```python
from build123d import *

# Parameters (mm, degrees)
SKETCH1_W           = 50
SKETCH1_H           = 60
BOSS_EXTRUDE1_DEPTH = 10
SKETCH2_R           = 1.5
CUT_EXTRUDE1_DEPTH  = 6
CUT_EXTRUDE2_REACH  = 41.509
SKETCH3_R           = 3
SKETCH5_W           = 25
SKETCH5_H           = 6
BOSS_EXTRUDE3_DEPTH = 30
CUT_EXTRUDE3_REACH  = 78.322
SKETCH6_W           = 22
SKETCH6_H           = 19.25
SKETCH7_R           = 1
CUT_EXTRUDE4_DEPTH  = 2.5
CUT_EXTRUDE5_REACH  = 75.602
SKETCH8_R           = 2
BOSS_EXTRUDE4_DEPTH = 5
CHAMFER1_SIZE       = 7.5
CHAMFER2_SIZE       = 10
CHAMFER4_SIZE       = 6.5
CHAMFER5_SIZE       = 4
CHAMFER6_SIZE       = 4
CHAMFER7_SIZE       = 2


# Some blends are built 0.0001 mm under size
with BuildPart() as part:
    # Sketch1 → Boss-Extrude1 (new body)
    with BuildSketch(Plane(origin=(0, 0, 0), x_dir=(1, 0, 0), z_dir=(0, 1, 0))):
        Rectangle(SKETCH1_W, SKETCH1_H)
    extrude(amount=BOSS_EXTRUDE1_DEPTH)

    # Sketch2 → Cut-Extrude1 (cut)
    with BuildSketch(Plane(origin=(0, 0, 0), x_dir=(1, 0, 0), z_dir=(0, 1, 0))):
        with Locations(Location((-21, 7.7, 0), (0, 0, 270))):
            Circle(SKETCH2_R)
        with Locations(Location((-21, -23, 0), (0, 0, 270))):
            Circle(SKETCH2_R)
        with Locations(Location((21, 7.7, 0), (0, 0, 270))):
            Circle(SKETCH2_R)
        with Locations(Location((21, -23, 0), (0, 0, 270))):
            Circle(SKETCH2_R)
    extrude(amount=CUT_EXTRUDE1_DEPTH, mode=Mode.SUBTRACT)

    # Sketch3 → Cut-Extrude2 (cut, up to next)
    with BuildSketch(Plane.XZ.offset(-6), mode=Mode.PRIVATE) as cut_extrude2_sk1:
        with Locations(Location((-21, 23, 0), (0, 0, 270))):
            Circle(SKETCH3_R)
    cut_extrude2_tool1 = extrude(cut_extrude2_sk1.sketch, amount=-CUT_EXTRUDE2_REACH, mode=Mode.PRIVATE) & part.part
    # Sketch3 → Cut-Extrude2 (cut, up to next)
    with BuildSketch(Plane.XZ.offset(-6), mode=Mode.PRIVATE) as cut_extrude2_sk2:
        with Locations(Location((21, 23, 0), (0, 0, 270))):
            Circle(SKETCH3_R)
    cut_extrude2_tool2 = extrude(cut_extrude2_sk2.sketch, amount=-CUT_EXTRUDE2_REACH, mode=Mode.PRIVATE) & part.part
    # Sketch3 → Cut-Extrude2 (cut, up to next)
    with BuildSketch(Plane.XZ.offset(-6), mode=Mode.PRIVATE) as cut_extrude2_sk3:
        with Locations(Location((21, -7.7, 0), (0, 0, 270))):
            Circle(SKETCH3_R)
    cut_extrude2_tool3 = extrude(cut_extrude2_sk3.sketch, amount=-CUT_EXTRUDE2_REACH, mode=Mode.PRIVATE) & part.part
    # Sketch3 → Cut-Extrude2 (cut, up to next)
    with BuildSketch(Plane.XZ.offset(-6), mode=Mode.PRIVATE) as cut_extrude2_sk4:
        with Locations(Location((-21, -7.7, 0), (0, 0, 270))):
            Circle(SKETCH3_R)
    cut_extrude2_tool4 = extrude(cut_extrude2_sk4.sketch, amount=-CUT_EXTRUDE2_REACH, mode=Mode.PRIVATE) & part.part
    add(cut_extrude2_tool1.solids().sort_by_distance((-21, 6, 23))[0], mode=Mode.SUBTRACT)
    add(cut_extrude2_tool2.solids().sort_by_distance((21, 6, 23))[0], mode=Mode.SUBTRACT)
    add(cut_extrude2_tool3.solids().sort_by_distance((21, 6, -7.7))[0], mode=Mode.SUBTRACT)
    add(cut_extrude2_tool4.solids().sort_by_distance((-21, 6, -7.7))[0], mode=Mode.SUBTRACT)

    # Sketch5 → Boss-Extrude3 (add)
    with BuildSketch(Plane(origin=(0, 10, 0), x_dir=(1, 0, 0), z_dir=(0, 1, 0))):
        with Locations((0, 27)):
            Rectangle(SKETCH5_W, SKETCH5_H)
    extrude(amount=BOSS_EXTRUDE3_DEPTH)

    # Sketch6 → Cut-Extrude3 (cut, up to next)
    with BuildSketch(Plane(origin=(0, 0, -30), x_dir=(-1, 0, 0), z_dir=(0, 0, -1)), mode=Mode.PRIVATE) as cut_extrude3_sk1:
        with Locations((0, 24.625)):
            Rectangle(SKETCH6_W, SKETCH6_H)
    cut_extrude3_tool1 = extrude(cut_extrude3_sk1.sketch, amount=-CUT_EXTRUDE3_REACH, mode=Mode.PRIVATE) & part.part
    add(cut_extrude3_tool1.solids().sort_by_distance((0, 24.625, -30))[0], mode=Mode.SUBTRACT)

    # Sketch7 → Cut-Extrude4 (cut)
    with BuildSketch(Plane.XY.offset(-24)):
        with Locations((10.25, 12.25)):
            Circle(SKETCH7_R)
        with Locations((-10.25, 12.25)):
            Circle(SKETCH7_R)
        with Locations((-10.25, 36.7)):
            Circle(SKETCH7_R)
        with Locations((10.25, 36.7)):
            Circle(SKETCH7_R)
    extrude(amount=-CUT_EXTRUDE4_DEPTH, mode=Mode.SUBTRACT)

    # Sketch8 → Cut-Extrude5 (cut, up to next)
    with BuildSketch(Plane.XY.offset(-26.5), mode=Mode.PRIVATE) as cut_extrude5_sk1:
        with Locations((-10.25, 36.7)):
            Circle(SKETCH8_R)
    cut_extrude5_tool1 = extrude(cut_extrude5_sk1.sketch, amount=-CUT_EXTRUDE5_REACH, mode=Mode.PRIVATE) & part.part
    # Sketch8 → Cut-Extrude5 (cut, up to next)
    with BuildSketch(Plane.XY.offset(-26.5), mode=Mode.PRIVATE) as cut_extrude5_sk2:
        with Locations((10.25, 36.7)):
            Circle(SKETCH8_R)
    cut_extrude5_tool2 = extrude(cut_extrude5_sk2.sketch, amount=-CUT_EXTRUDE5_REACH, mode=Mode.PRIVATE) & part.part
    # Sketch8 → Cut-Extrude5 (cut, up to next)
    with BuildSketch(Plane.XY.offset(-26.5), mode=Mode.PRIVATE) as cut_extrude5_sk3:
        with Locations((10.25, 12.25)):
            Circle(SKETCH8_R)
    cut_extrude5_tool3 = extrude(cut_extrude5_sk3.sketch, amount=-CUT_EXTRUDE5_REACH, mode=Mode.PRIVATE) & part.part
    # Sketch8 → Cut-Extrude5 (cut, up to next)
    with BuildSketch(Plane.XY.offset(-26.5), mode=Mode.PRIVATE) as cut_extrude5_sk4:
        with Locations((-10.25, 12.25)):
            Circle(SKETCH8_R)
    cut_extrude5_tool4 = extrude(cut_extrude5_sk4.sketch, amount=-CUT_EXTRUDE5_REACH, mode=Mode.PRIVATE) & part.part
    add(cut_extrude5_tool1.solids().sort_by_distance((-10.25, 36.7, -26.5))[0], mode=Mode.SUBTRACT)
    add(cut_extrude5_tool2.solids().sort_by_distance((10.25, 36.7, -26.5))[0], mode=Mode.SUBTRACT)
    add(cut_extrude5_tool3.solids().sort_by_distance((10.25, 12.25, -26.5))[0], mode=Mode.SUBTRACT)
    add(cut_extrude5_tool4.solids().sort_by_distance((-10.25, 12.25, -26.5))[0], mode=Mode.SUBTRACT)

    # Sketch9 → Boss-Extrude4 (add)
    with BuildSketch(Plane(origin=(12.5, 0, 0), x_dir=(0, 0, -1), z_dir=(1, 0, 0))):
        Polygon((30, 40), (24, 40), (-6, 10), (30, 10), align=None)
    boss_extrude4 = extrude(amount=BOSS_EXTRUDE4_DEPTH)

    # Mirror1: Boss-Extrude4 across plane
    add(boss_extrude4.mirror(Plane(origin=(0, 0, 0), x_dir=(0, 0, 1), z_dir=(1, 0, 0))))

    # Chamfer1
    # the kernel refuses this chamfer: 7.5 mm, written as the material it adds along each edge
    with BuildSketch(Plane(origin=(17.5, 10, 25.28762241), x_dir=(-0.02749587661058632, 0.9996219169112968, 0), z_dir=(0, 0, -1))) as chamfer1_piece_1_section:
        Polygon((CHAMFER1_SIZE * 0.999621916911, CHAMFER1_SIZE * 0.0274958766106), (-CHAMFER1_SIZE * 0.0274958766106, CHAMFER1_SIZE * 0.999621916911), (0, 0), align=None)
    chamfer1_piece_1 = extrude(amount=55.28762241, mode=Mode.PRIVATE)
    chamfer1_piece_1 = split(chamfer1_piece_1, bisect_by=Plane(origin=(19.963540821, 21.141387269, -5.141387269), z_dir=(0, -0.7071067811865512, -0.7071067811865438)), keep=Keep.TOP, mode=Mode.PRIVATE)
    chamfer1_piece_1 = chamfer1_piece_1 - Plane(origin=(21, 12.394681138, -7.7), x_dir=(0, 0, -1), z_dir=(0, -1, 0)) * Cylinder(3, 141, mode=Mode.PRIVATE)
    chamfer1_piece_1 = split(chamfer1_piece_1, bisect_by=Plane(origin=(25, 12.394681138, -13.888093401), z_dir=(-1, 0, 0)), keep=Keep.TOP, mode=Mode.PRIVATE)
    add(chamfer1_piece_1)
    with BuildSketch(Plane(origin=(-17.5, 10, 25.28762241), x_dir=(0.02749587661058632, 0.9996219169112968, 0), z_dir=(0, 0, -1))) as chamfer1_piece_2_section:
        Polygon((CHAMFER1_SIZE * 0.999621916911, -CHAMFER1_SIZE * 0.0274958766106), (-CHAMFER1_SIZE * 0.0274958766106, -CHAMFER1_SIZE * 0.999621916911), (0, 0), align=None)
    chamfer1_piece_2 = extrude(amount=55.28762241, mode=Mode.PRIVATE)
    chamfer1_piece_2 = split(chamfer1_piece_2, bisect_by=Plane(origin=(-19.963548268, 21.141369022, -5.141369022), z_dir=(0, -0.7071067811865512, -0.7071067811865438)), keep=Keep.TOP, mode=Mode.PRIVATE)
    chamfer1_piece_2 = chamfer1_piece_2 - Plane(origin=(-21, 12.394672857, -7.7), x_dir=(0, 0, -1), z_dir=(0, -1, 0)) * Cylinder(3, 141, mode=Mode.PRIVATE)
    chamfer1_piece_2 = split(chamfer1_piece_2, bisect_by=Plane(origin=(-25, 12.394672857, -13.888065186), z_dir=(1, 0, 0)), keep=Keep.TOP, mode=Mode.PRIVATE)
    add(chamfer1_piece_2)

    # Chamfer2
    chamfer2_edges = [part.edges().sort_by_distance(p)[0] for p in [
        (-25, 5, -30),
        (25, 5, -30),
    ]]
    chamfer(chamfer2_edges, length=CHAMFER2_SIZE)

    # Chamfer4
    chamfer4_edges = [part.edges().sort_by_distance(p)[0] for p in [
        (0, 0, -30),
    ]]
    chamfer(chamfer4_edges, length=CHAMFER4_SIZE)

    # Chamfer5
    chamfer5_edges = [part.edges().sort_by_distance(p)[0] for p in [
        (17.5, 40, -25.75),
        (-17.5, 40, -25.75),
    ]]
    chamfer(chamfer5_edges, length=CHAMFER5_SIZE)

    # Chamfer6
    chamfer6_edges = [part.edges().sort_by_distance(p)[0] for p in [
        (0, 10, 30),
    ]]
    chamfer(chamfer6_edges, length=CHAMFER6_SIZE - 0.0001)  # a hair under: the kernel refuses the full size

    # Chamfer7
    chamfer7_edges = [part.edges().sort_by_distance(p)[0] for p in [
        (-11, 34.25, -27),
        (-11, 15, -27),
        (11, 15, -27),
        (11, 34.25, -27),
    ]]
    chamfer(chamfer7_edges, length=CHAMFER7_SIZE)


solid = part.part
```
Can you work these out from the model? Positions are in its coordinate system, mm. A direction names the side the tool comes from. Give positions to 0.01 mm unless a question says otherwise; leave off trailing zeros. Loops run counter-clockwise (first coordinate to the right, second up) from the corner with the lowest first, then second, coordinate; pieces in that order, holes last. Notation, with made-up numbers: M 55,68.5 L 98,68.5 A26 cw 98,107.5 Z; hole C 8.5,45 d11. An arc over 180 degrees is marked long. Use CSV: the item, a comma, the result in double quotes. Start each with the question number.
1. Imagine slicing it at A-A, the plane y = 27.5. Write out the boundary of the cut face in (x, z), plus the area to 3 significant figures.
2. For P1, Ø6.5, axis at y = 25, z = -26.5, coming from the -X side; P2, Ø2.5, axis at x = 10.25, y = 36.7, coming from the -Z side; P3, Ø6, axis at y = 16, z = -13, coming from the +X side, each with a flat end and sliding along its axis, tell me the tip position at first contact or that it passes through.
3. If we mould it in two halves opening along Z, with no side actions, what happens to faces 1 (the face through (-10, 38, -26.5)), 2 (the face through (-18.026, 10.228, -7.309)), 3 (the face through (0, 15, -27)), 4 (the face through (-19.513, 2.958, -7.895))? For each: released by +Z, released by -Z, zero draft, split by the parting line, or undercut.
4. Imagine slicing it at D-D, the plane y = 33.5. Write out the boundary of the cut face in (x, z), plus the area to 3 significant figures.
5. Imagine slicing it at C-C, the plane z = 23. Write out the boundary of the cut face in (x, y), plus the area to 3 significant figures.
6. Imagine slicing it at B-B, the plane x = 7.5. Write out the boundary of the cut face in (y, z).
7. On a 3-axis mill with a long thin cutter (end or side, diameter ignored), from which of +Z, -Z, +X, -X, +Y, -Y can I reach the whole of each face in a straight line? I mean faces 5 (the face through (0, 10, 6)), 6 (the face through (-17.5, 25, -17)), 7 (the face through (-10.01, 33.24, -27.04)), 8 (the face through (9, 12, -26.5)). Say none if no direction works.
8. If I drill on L1, parallel to X at y = 35, z = -23.5; L2, parallel to X at y = 2, z = 23; L3, parallel to Z at x = -8.5, y = 14.5, over which ranges is the centre line in solid material (lowest first)?
Response values:
1,outline,"M -17.5,-27.5 L -15,-30 L -11,-30 L -11,-24 L -12.5,-24 L -12.5,-11.5 L -17.5,-11.5 Z; M 11,-30 L 15,-30 L 17.5,-27.5 L 17.5,-11.5 L 12.5,-11.5 L 12.5,-24 L 11,-24 Z"
1,area,"197 mm^2"
2,P1,"x = -17.5"
2,P2,"z = -26.5"
2,P3,"x = 22"
3,face 1,"released by -Z"
3,face 2,"undercut"
3,face 3,"zero draft"
3,face 4,"undercut"
4,outline,"M -17.5,-27.5 L -15,-30 L -9.75,-30 L -9.75,-24 L -12.5,-24 L -12.5,-17.5 L -17.5,-17.5 Z; M 9.75,-30 L 15,-30 L 17.5,-27.5 L 17.5,-17.5 L 12.5,-17.5 L 12.5,-24 L 9.75,-24 Z"
4,area,"152 mm^2"
5,outline,"M -25,0 L -22.5,0 L -22.5,6 L -24,6 L -24,10 L -25,10 Z; M -19.5,0 L 19.5,0 L 19.5,6 L 18,6 L 18,10 L -18,10 L -18,6 L -19.5,6 Z; M 22.5,0 L 25,0 L 25,10 L 24,10 L 24,6 L 22.5,6 Z"
5,area,"416 mm^2"
6,outline,"M 0,-23.5 L 6.5,-30 L 15,-30 L 15,-24 L 10,-24 L 10,26 L 6,30 L 0,30 Z; M 34.25,-30 L 40,-30 L 40,-24 L 34.25,-24 Z"
7,face 5,"+Z, +Y"
7,face 6,"+Z, -Z, -X, +Y"
7,face 7,"+Z, -Z"
7,face 8,"-Z"
8,L1,"-17.5 to -12.5, 12.5 to 17.5"
8,L2,"-25 to -22.5, -19.5 to 19.5, 22.5 to 25"
8,L3,"-30 to -24"
